from build123d import *

# Parameters (mm, degrees)
F0_R     = 7.5
F0_R_2   = 4.55
F1_DEPTH = 10


with BuildPart() as f1:
    # F0 (on Top) → F1 (new body)
    with BuildSketch(Plane.XY):
        Circle(F0_R)
        Circle(F0_R_2, mode=Mode.SUBTRACT)
    extrude(amount=F1_DEPTH)

    # F2 (on Front) → F4 (revolve, cut)
    with BuildSketch(Plane.XZ):
        Polygon((7.5, 1.5), (4.55, 0), (7.5, 0), align=None)
    revolve(axis=Axis((0, 0, 29.497309), (0, 0, 1)), mode=Mode.SUBTRACT)

    # F5 (on Front) → F6 (revolve, cut)
    with BuildSketch(Plane.XZ):
        Polygon((7.5, 10), (4.55, 10), (7.5, 8.5), align=None)
    revolve(axis=Axis((0, 0, 0), (0, 0, -1)), mode=Mode.SUBTRACT)


solid = f1.part
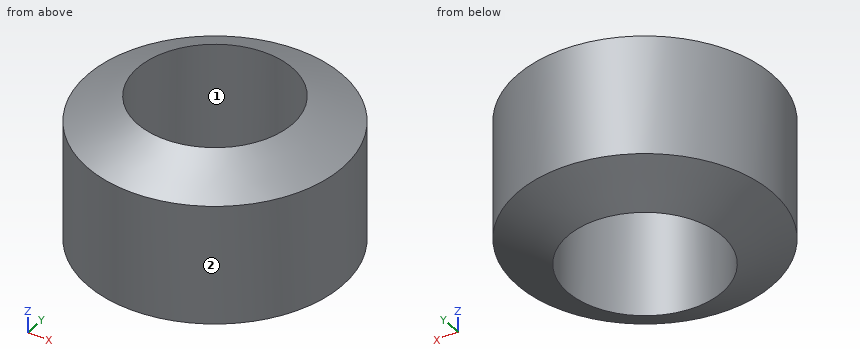
The listing builds one solid part. Answer for the finished solid, in the listing's coordinates (mm). Face numbers are marked on the shaded views. Coordinates: 2 decimals unless noted, no trailing zeros. Order: outer loops, then holes, each group sorted by start corner. A loop starts at its lowest first (then second) coordinate and runs counter-clockwise, first axis right, second up.
Q1. Given P1, Ø3, axis at x = -3.5, z = 4, coming from the +Y side; P2, Ø1, axis at y = 5.5, z = 6, coming from the +X side, each flat-ended and moving along its own axis, determine where each tip first touches the part or whether it passes through.
Q2. A cutting plane is placed at A-A, the plane x = 0. Write down the section's boundary in (y, z), and give its area (4 significant figures).
Q3. A cutting plane is placed at C-C, the plane z = 7. Write down the section's boundary in (x, y).
Q4. For a pull along X with two mould halves and no side action, classify the marked faces 1 and 2 as pulls with the +X half, pulls with the -X half, needs draft (parallel to the pull), parting line crosses it, or undercut.
Q5. Consider line 1 (Y direction, x = 0, z = 6.5); line 2 (X direction, y = -3.5, z = 8.25); line 3 (X direction, y = 2, z = 5.5). Determine where each line is inside the solid, lowest interval first.
Answers follow:
1. P1: stops at y = 7.23
1. P2: stops at x = 5.59
2. outline: (-7.5, 1.5) - (-4.55, 0) - (-4.55, 10) - (-7.5, 8.5) - close; (4.55, 0) - (7.5, 1.5) - (7.5, 8.5) - (4.55, 10) - close
2. area: 50.15 mm2
3. outline: circle Ø15 at (0, 0); hole circle Ø9.1 at (0, 0)
4. face 1: undercut
4. face 2: parting line crosses it
5. line 1: y = -7.5 to -4.55, 4.55 to 7.5
5. line 2: x = -6.63 to -2.91, 2.91 to 6.63
5. line 3: x = -7.23 to -4.09, 4.09 to 7.23
